Verification items for the finished model (mm, model axes). Face numbers are marked on the shaded views. A direction names the side the tool comes from. Round coordinates to 2 decimals unless told otherwise and drop trailing zeros. Write each loop counter-clockwise with the first axis right and the second up, starting at its lowest first coordinate (ties: lowest second). Pieces come first, ordered by that corner, then holes. Notation, with made-up numbers: (22.25, 8.25) -> (37.25, 8.25) arc R21 ccw to (37.25, 36.25) -> close; hole circle Ø3 at (-19, -2.5). An arc over 180 degrees is marked (long way). Use CSV: the item, a comma, the result in double quotes.
```python
from build123d import *

# Parameters (mm, degrees)
BOSS_EXTRUDE1_DEPTH  = 2
BOSS_EXTRUDE2_DEPTH  = 2
MIRROR2_COPY_1_DEPTH = 2
STOPPER_DEPTH        = 2
STOPPER_DEBURS_SIZE  = 0.2


with BuildPart() as part:
    # Sketch1 → Boss-Extrude1 (new body)
    with BuildSketch(Plane.XY):
        Polygon((-11.5, 4), (11.5, 4), (11.5, -4), (5, -4), (5, 2), (-5, 2), (-5, -4), (-11.5, -4), align=None)
    extrude(amount=-BOSS_EXTRUDE1_DEPTH)

    # Sketch2 → Boss-Extrude2 (add)
    with BuildSketch(Plane.XY):
        with BuildLine():
            Line((11.5, -3.5), (11.5, 1))
            Line((11.5, 1), (11.328427125, 1))
            ThreePointArc((11.328427125, 1), (10.601328603, 0.855371112), (9.98492424, 0.443502884))
            Line((9.98492424, 0.443502884), (9.6, 0.058578644))
            Line((9.6, 0.058578644), (9.6, -2.558578644))
            Line((9.6, -2.558578644), (9.98492424, -2.943502884))
            ThreePointArc((9.98492424, -2.943502884), (10.601328603, -3.355371112), (11.328427125, -3.5))
            Line((11.328427125, -3.5), (11.5, -3.5))
        make_face()
    boss_extrude2 = extrude(amount=BOSS_EXTRUDE2_DEPTH)

    # Mirror1: Boss-Extrude2 across plane
    add(boss_extrude2.mirror(Plane(origin=(8.25, 0, 0), x_dir=(0, 0, 1), z_dir=(1, 0, 0))))

    # Mirror2: Boss-Extrude2 across plane
    add(boss_extrude2.mirror(Plane(origin=(0, 0, 0), x_dir=(0, 0, 1), z_dir=(1, 0, 0))))

    # Mirror2 copy 1 sketch → Mirror2 copy 1 (add)
    with BuildSketch(Plane(origin=(-16.5, 0, 0), x_dir=(1, 0, 0), z_dir=(0, 0, 1))):
        with BuildLine():
            Line((11.5, -3.5), (11.5, 1))
            Line((11.5, 1), (11.328427125, 1))
            ThreePointArc((11.328427125, 1), (10.601328603, 0.855371112), (9.98492424, 0.443502884))
            Line((9.98492424, 0.443502884), (9.6, 0.058578644))
            Line((9.6, 0.058578644), (9.6, -2.558578644))
            Line((9.6, -2.558578644), (9.98492424, -2.943502884))
            ThreePointArc((9.98492424, -2.943502884), (10.601328603, -3.355371112), (11.328427125, -3.5))
            Line((11.328427125, -3.5), (11.5, -3.5))
        make_face()
    extrude(amount=MIRROR2_COPY_1_DEPTH)

    # Sketch4 → Stopper (add)
    with BuildSketch(Plane(origin=(0, 0, -2), x_dir=(-1, 0, 0), z_dir=(0, 0, -1))):
        Polygon((11.5, -4), (14, -4), (14, 5.65), (-14, 5.65), (-14, -4), (-11.5, -4), (-5, -4), (-5, 2), (5, 2), (5, -4), align=None)
    extrude(amount=STOPPER_DEPTH)

    # Stopper Deburs
    stopper_deburs_edges = [part.edges().sort_by_distance(p)[0] for p in [
        (-11.414213562, 1, 2),
        (-11.414213562, -3.5, 2),
        (-10.601328603, -3.355371112, 2),
        (-14, -4, -3),
        (-14, 5.65, -3),
        (14, 5.65, -3),
        (14, -4, -3),
        (-9.5, -4, -4),
        (-14, 0.825, -4),
        (0, 5.65, -4),
        (14, 0.825, -4),
        (9.5, -4, -4),
        (5, -1, -4),
        (0, 2, -4),
        (-5, -1, -4),
        (-11.5, 4, -1),
        (11.5, 4, -1),
        (11.5, -4, -1),
        (5, -4, -2),
        (-5, -4, -2),
        (-11.5, -4, -1),
        (9.79246212, -2.751040764, 2),
        (10.601328603, -3.355371112, 2),
        (11.414213562, -3.5, 2),
        (11.414213562, 1, 2),
        (10.601328603, 0.855371112, 2),
        (9.79246212, 0.251040764, 2),
        (9.6, -1.25, 2),
        (6.70753788, -2.751040764, 2),
        (6.9, -1.25, 2),
        (6.70753788, 0.251040764, 2),
        (5.898671397, 0.855371112, 2),
        (5.085786438, 1, 2),
        (5.085786438, -3.5, 2),
        (5.898671397, -3.355371112, 2),
        (-6.70753788, -2.751040764, 2),
        (-5.898671397, -3.355371112, 2),
        (-5.085786438, -3.5, 2),
        (-5.085786438, 1, 2),
        (-5.898671397, 0.855371112, 2),
        (-6.70753788, 0.251040764, 2),
        (-6.9, -1.25, 2),
        (-9.79246212, -2.751040764, 2),
        (-9.6, -1.25, 2),
        (-9.79246212, 0.251040764, 2),
        (-10.601328603, 0.855371112, 2),
    ]]
    chamfer(stopper_deburs_edges, length=STOPPER_DEBURS_SIZE)


solid = part.part
```
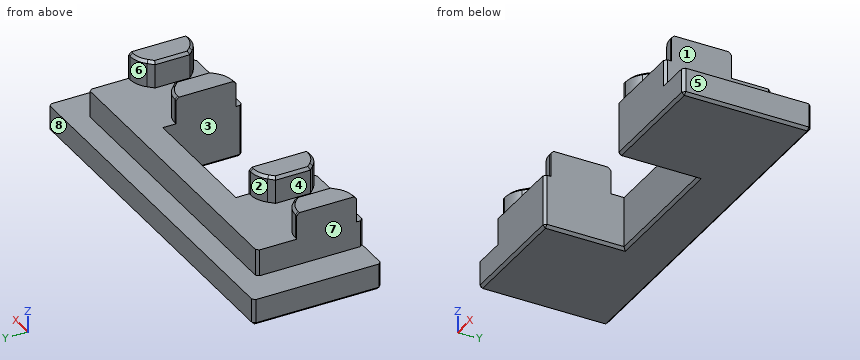
Q1. Section check B-B (z = 1). State how many separate pieces and enclosed holes the cut face has, plus the area to 3 significant figures.
Filled in:
separate pieces,"4"
enclosed holes,"0"
area,"30.0 mm²"
Q2. Section check C-C (x = 8.25). Record the cut outline in (y, z), plus the area to 3 significant figures.
Filled in:
outline,"(-4, -3.8) -> (-3.8, -4) -> (5.45, -4) -> (5.65, -3.8) -> (5.65, -2) -> (4, -2) -> (4, 0) -> (-4, 0) -> close"
area,"35.3 mm²"
Q3. Section check D-D (z = -3.5). Record the cut outline in (x, y).
Filled in:
outline,"(-14, -3.8) -> (-13.8, -4) -> (-5.2, -4) -> (-5, -3.8) -> (-5, 2) -> (5, 2) -> (5, -3.8) -> (5.2, -4) -> (13.8, -4) -> (14, -3.8) -> (14, 5.45) -> (13.8, 5.65) -> (-13.8, 5.65) -> (-14, 5.45) -> close"
Q4. Go/stop test with flat-tipped pins: P1, Ø2, axis at y = 1.5, z = 0, coming from the +X side; P2, Ø1.4, axis at y = -1, z = 1, coming from the -X side; P3, Ø1.1, axis at x = -1, z = -2.5, coming from the -Y side. Record where each tip stops, or that it passes through.
Filled in:
P1,"x = 11.5"
P2,"x = -11.5"
P3,"y = 2"
Q5. Mould release check, pull along X, two halves, no side actions. Record for the marked faces 5, 6, 7 and 8: released by +X, released by -X, zero draft, split by the parting line, or undercut.
Filled in:
face 5,"released by +X"
face 6,"undercut"
face 7,"released by -X"
face 8,"zero draft"
Q6. Access from +Z, -Z, +X, -X, +Y, -Y to the whole of each face (thin tool, end or side, straight path). Record for the marked faces 1, 2, 3 and 4.
Filled in:
face 1,"+Z, +X, +Y, -Y"
face 2,"+Z, +Y"
face 3,"+Z, -Z, -Y"
face 4,"+Z, +Y, -Y"
Q7. Material ranges on L1, parallel to X at y = -1, z = 1.25; L2, parallel to X at y = 0, z = -3.5; L3, parallel to X at y = -0.75, z = -0.75, recorded low to high.
Filled in:
L1,"-11.5 to -9.6, -6.9 to -5, 5 to 6.9, 9.6 to 11.5"
L2,"-14 to -5, 5 to 14"
L3,"-11.5 to -5, 5 to 11.5"
Q8. Section check A-A (y = -1.25). Record the cut outline in (x, z).
Filled in:
outline,"(-14, -3.8) -> (-13.8, -4) -> (-5.2, -4) -> (-5, -3.8) -> (-5, 2) -> (-6.7, 2) -> (-6.9, 1.8) -> (-6.9, 0) -> (-9.6, 0) -> (-9.6, 1.8) -> (-9.8, 2) -> (-11.5, 2) -> (-11.5, -2) -> (-14, -2) -> close; (5, -3.8) -> (5.2, -4) -> (13.8, -4) -> (14, -3.8) -> (14, -2) -> (11.5, -2) -> (11.5, 2) -> (9.8, 2) -> (9.6, 1.8) -> (9.6, 0) -> (6.9, 0) -> (6.9, 1.8) -> (6.7, 2) -> (5, 2) -> close"
